Autodesk Fusion 360 part; units mm, degrees
sketch "Sketch1" plane through (0, 0, 0) normal (0, 1, 0) x (1, 0, 0)
  circle A0 centre (0, 0) radius 22.375
  circle A1 centre (0, 0) radius 25
  dimension "d1" = 44.75
  dimension "d2" = 50
sketch "Sketch2" plane through (0, 0, 0) normal (0, 0, 1) x (1, 0, 0)
extrude "Extrude1" add sketch "Sketch1" along normal blind 3
sketch "Sketch3" plane through (0, 0, 0) normal (0, 0, 1) x (1, 0, 0)
  line L0 (18, 0) -> (18, -6)
  line L1 (25, 0) -> (25, -6)
  line L2 (18, -6) -> (25, -6)
  line L3 (18, 0) -> (25, 0)
  line L4 (18, -6) -> (25, -6)
  circle A0 centre (17.7502, -1.1354) radius 5.5639
  circle A1 centre (17.685, 1.409) radius 7.4494
  dimension "d9" = 18
  dimension "d10" = 25
  dimension "d11" = 6
  dimension "d12" = 6
sketch "Sketch4" plane through (0, 0, 0) normal (0, 0, 1) x (1, 0, 0)
sketch "Sketch5" plane through (0, 0, 0) normal (0, 0, 1) x (1, 0, 0)
  line L0 (-15, -0.0108) -> (15, -0.0108)
  line L1 (15, -0.0108) -> (15, -9.5655)
  line L2 (15, -9.5655) -> (-15, -9.5655)
  line L3 (-15, -9.5655) -> (-15, -0.0108)
  dimension "d14" = 30
  dimension "d15" = 15
sketch "Sketch6" plane through (0, 3, 0) normal (0, 1, 0) x (-1, 0, 0)
  circle A0 centre (0, 0) radius 22.375
  circle A1 centre (0, 0) radius 25
sketch "Sketch7" plane through (0, 0, 0) normal (1, 0, 0) x (0, 0, -1)
  line L0 (-3.5, 2.9971) -> (3.5, 2.9971)
  line L1 (3.5, 2.9971) -> (3.5, -7)
  line L2 (3.5, -7) -> (-3.5, -7)
  line L3 (-3.5, -7) -> (-3.5, 2.9971)
  point P0 (0, 1.409)
  dimension "d20" = 7
  dimension "d26" = 3.5
sketch "Sketch8" plane through (0, 0, 0) normal (0, 0, 1) x (1, 0, 0)
sketch "Sketch9" plane through (0, 3, 0) normal (0, 1, 0) x (-1, 0, 0)
extrude "Extrude4" cut sketch "Sketch7" along normal blind 25
extrude "Extrude5" cut sketch "Sketch5" along normal blind 32 and the other way blind 36
sketch "Sketch10" plane through (0, 3, 0) normal (0, 1, 0) x (-1, 0, 0)
  line L0 (7.5, -33) -> (-7.5, -33)
  line L1 (-7.5, -33) -> (-7.5, -23)
  line L2 (-7.5, -23) -> (7.5, -23)
  line L3 (7.5, -23) -> (7.5, -33)
  circle A0 centre (3.75, -28) radius 2.6
  circle A1 centre (-3.75, -28) radius 2.6
  dimension "d33" = 15
  dimension "d34" = 7.5
  dimension "d35" = 5.2
  dimension "d36" = 5.2
  dimension "d37" = 10
  dimension "d38" = 23
  dimension "d39" = 3.75
  dimension "d40" = 3.75
revolve "Revolve4" add sketch "Sketch3" angle 360 about axis through (0, 1.75, 0) along (0, 1, 0) contours L3 A0 A1 picked at (24.3244, -0.4805)
extrude "Extrude9" cut sketch "Sketch5" along normal blind 42 and the other way blind 47
extrude "Extrude10" cut sketch "Sketch7" along normal blind 53
sketch "Sketch11" plane through (0, 0, 0) normal (0, 0, 1) x (1, 0, 0)
sketch "Sketch12" plane through (0, 0, 0) normal (0, 1, 0) x (1, 0, 0)
extrude "Extrude11" add sketch "Sketch10" against normal blind 3
extrude "Extrude12" add 1 faces at (1.0571, 3, -32.1783) along direction (0, 1, 0) blind 1
sketch "Sketch13" plane through (0, 0, 0) normal (0, 0, 1) x (1, 0, 0)
sketch "Sketch14" plane through (0, 0, 0) normal (1, 0, 0) x (0, 0, -1)
sketch "Sketch15" plane through (7.5, 0, 0) normal (1, 0, 0) x (0, 0, -1)
  line L0 (23.8485, 4) -> (23.8485, 0)
  line L1 (23.8485, 0) -> (33, 0)
  line L2 (33, 0) -> (33, 4)
  line L3 (33, 4) -> (23.8485, 4)
sketch "Sketch16" plane through (0, 0, 0) normal (1, 0, 0) x (0, 0, -1)
equation "d10 = ( 50 / 2 ) * 1 mm"
equation "d39 = ( 7.5 / 2 ) * 1 mm"
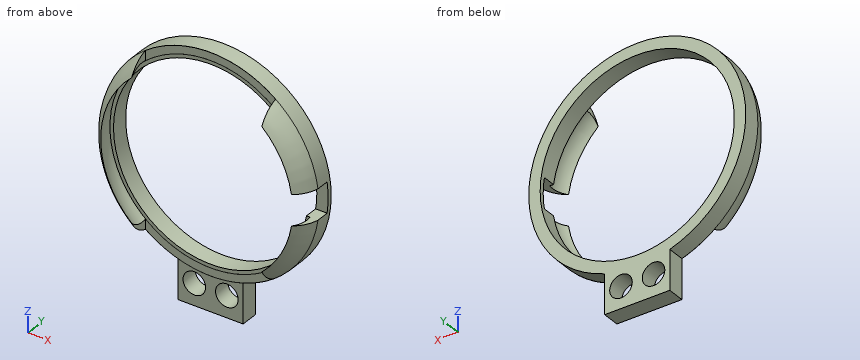
Source: CAD feature listing. Evaluate the final solid. Frame: model axes, mm. Give positions to 0.01 mm unless a question says otherwise; leave off trailing zeros. Loops run counter-clockwise (first coordinate to the right, second up) from the corner with the lowest first, then second, coordinate; pieces in that order, holes last. Notation, with made-up numbers: (63, -25.75) -> (109, -25.75) arc R33 ccw to (109, 8.25) -> close; hole circle Ø8 at (8.5, 19.25). An arc over 180 degrees is marked (long way). Use a Markdown table: item, result. Add a question column.
1) Line query: line 1 along Z through (x, y) = (0, 1.65) (3 decimals); line 2 along Z through (x, y) = (3.75, 3); line 3 along Z through (x, y) = (-2, 2.25). Output: solid intervals per line, ascending. Write a range as [from, to].
2) Section query D-D, the plane y = 1.5. Return the cut outline in (x, z) (3 decimals), then the cut area to 3 significant figures.
3) Section query A-A, the plane x = 0. Return the cut outline in (y, z) (3 decimals), then the cut area to 3 significant figures.
4) Section query B-B, the plane y = -2.5. Return the cut outline in (x, z), then the cut area to 3 significant figures.
5) First-contact query: pin 1 (6 mm diameter, centred on x = -2.5, z = 20.5, fed in from -Y); pin 2 (1.5 mm diameter, centred on x = 22.5, y = -2, fed in from +Z); pin 3 (3 mm diameter, centred on y = -2.5, z = -18.5, fed in from -X); pin 4 (4.5 mm diameter, centred on x = -3.75, z = -28, fed in from -Y). Flat tips, straight axial feed; report the tip coordinate or a pass-through.
6) Section query C-C, the plane z = 0. Return the cut outline in (x, y) (3 decimals).
Numbers:
| question | item | result |
|---|---|---|
| 1 | line 1 | z = [-33, -22.375], [22.375, 25] |
| 1 | line 2 | z = [-33, -30.6], [-25.4, -22.06], [22.06, 24.72] |
| 1 | line 3 | z = [-33, -29.92], [-26.08, -22.29], [22.29, 24.92] |
| 2 | outline | (-7.5, -33) -> (7.5, -33) -> (7.5, -23.848) arc R25 ccw to (24.754, -3.5) -> (22.1, -3.5) arc R22.375 cw (long way) to (22.1, 3.5) -> (24.754, 3.5) arc R25 ccw (long way) to (-7.5, -23.848) -> close; hole circle Ø5.2 at (-3.75, -28); hole circle Ø5.2 at (3.75, -28) |
| 2 | area | 455 mm2 |
| 3 | outline | (-0.011, -24.998) arc R7.449 ccw to (0, -25) -> (0, -33) -> (4, -33) -> (4, -22.375) -> (0, -22.375) -> (0, -23.197) arc R5.564 cw to (-0.011, -23.199) -> close; (-0.011, 23.199) arc R5.564 cw to (0, 23.197) -> (0, 22.375) -> (4, 22.375) -> (4, 25) -> (0, 25) arc R7.449 ccw to (-0.011, 24.998) -> close |
| 3 | area | 53.0 mm2 |
| 4 | outline | (-15, -18.77) -> (-15, -17.63) arc R23.14 cw to (-15, 17.63) -> (-15, 18.77) arc R24.03 ccw to start; (15, -18.77) arc R24.03 ccw to (23.77, -3.5) -> (22.88, -3.5) arc R23.14 cw to (15, -17.63) -> close; (15, 17.63) arc R23.14 cw to (22.88, 3.5) -> (23.77, 3.5) arc R24.03 ccw to (15, 18.77) -> close |
| 4 | area | 67.2 mm2 |
| 5 | pin 1 | stops at y = -0.01 |
| 5 | pin 2 | stops at z = 11.06 |
| 5 | pin 3 | stops at x = -17.35 |
| 5 | pin 4 | passes through |
| 6 | outline | (-25, 0) arc R7.449 ccw to (-22.126, -4.572) arc R5.564 cw to (-23.197, 0) -> (-22.375, 0) -> (-22.375, 4) -> (-25, 4) -> close; (22.375, 2.997) -> (25, 2.997) -> (25, 4) -> (22.375, 4) -> close |
